Autodesk Inventor part; units mm, degrees
ref_plane "YZ Plane" through (0, 0, 0) normal (1, 0, 0) x (0, 1, 0)
ref_plane "XZ Plane" through (0, 0, 0) normal (0, 1, 0) x (-1, 0, 0)
ref_plane "XY Plane" through (0, 0, 0) normal (0, 0, 1) x (1, 0, 0)
sketch "Sketch1" plane through (0, 0, 0) normal (0, 1, 0) x (-1, 0, 0)
  circle A0 centre (0, 0) radius 90
  line L0 (-25, 120) -> (-25, 60)
  line L1 (-25, 60) -> (-145, 60)
  line L2 (-145, 60) -> (-145, 120)
  line L3 (-145, 120) -> (-25, 120)
  line L4 (-25, 90) -> (0, 90)
  line L5 (-65, 131) -> (-38.5, 131)
  line L6 (-38.5, 131) -> (-38.5, 49)
  line L7 (-38.5, 49) -> (-65, 49)
  line L8 (-65, 49) -> (-65, 131)
  line L9 (-38.5, 90) -> (-25, 90) construction
  circle A1 centre (0, 0) radius 150
  line L10 (-25, 30) -> (25, 30)
  line L11 (25, 30) -> (25, 150)
  line L12 (25, 150) -> (-25, 150)
  line L13 (-25, 150) -> (-25, 30)
  line L14 (-25, 30) -> (25, 150) construction
  line L15 (25, 30) -> (-25, 150) construction
  point P0 (-65, 62.2495)
  point P1 (-65, 60)
  point P2 (-67.082, 60)
  point P3 (25, 147.902)
  point P4 (-25, 147.902)
  dimension "d0" = 180
  dimension "d1" = 25
  dimension "d2" = 60
  dimension "d3" = 120
  dimension "d4" = 82
  dimension "d5" = 26.5
  dimension "d7" = 38.5
  dimension "d8" = 300
  dimension "d18" = 50
  dimension "d19" = 120
extrude "Extrusion1" add sketch "Sketch1" against normal blind 6 contours A0 L1 L8 L7 L6 L13 L10 L11 | A0 L11 A1 L1 | L11 L10 L13 L0 A0 | A0 L4 L0 L13 A1 L11 | L1 A1 L3 L8 A0 | A0 L8 L1 | A0 L0 L4 | L8 L3 L6 A0 | A0 L6 L1 L8 | L1 L6 L7 L8 | L0 L1 L6 A0 | A0 L6 L3 L0 | L8 L5 L6 L3 | L3 A1 L13 L6 L5 L8
hole "Hole1" at (65, 0, 131) at (38.5, 0, 131) at (65, 0, 49) at (38.5, 0, 49) direction (0, -1, 0) diameter 5.6 end through all
extrude "Extrusion2" cut sketch "Sketch1" against normal blind 6 contours L11 L10 L13 L0 A0 | A0 L4 L0 L13 A1 L11 | A0 L0 L4
pattern_circular "Circular Pattern1" count 3 over 360 about axis through (0, 0, 0) along (0, -1, 0) of "Hole1", "Extrusion2"
properties part number "TempPart1"
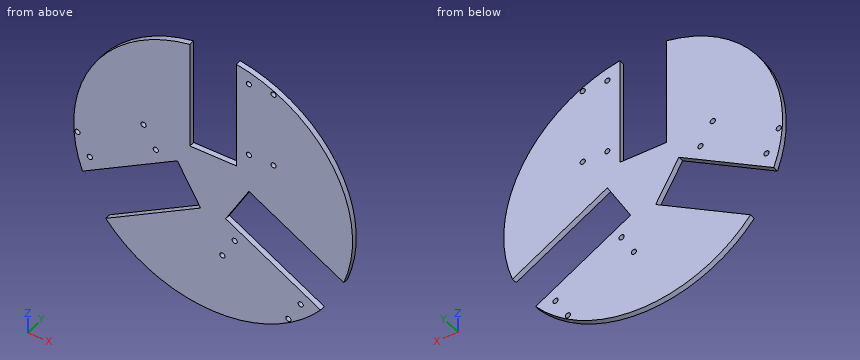
Geometry check sheet. Reference: the model listing, model coordinates, mm. Give positions to 0.01 mm unless a question says otherwise; leave off trailing zeros. Write each loop counter-clockwise with the first axis right and the second up, starting at its lowest first coordinate (ties: lowest second). Pieces come first, ordered by that corner, then holes. Notation, with made-up numbers: (60.25, -15) - (83.25, -15) arc R27 cw to (83.25, 13) - close; hole circle Ø3 at (-5.5, -20). An arc over 180 degrees is marked (long way). Use a Markdown table: item, result.
Q1. Section check A-A, the plane z = 77.5. Enter the section's corners in (x, y).
Computed:
| item | result |
|---|---|
| outline | (-128.43, -6) - (-25, -6) - (-25, 0) - (-128.43, 0) - close; (25, -6) - (128.43, -6) - (128.43, 0) - (25, 0) - close |
Q2. Thickness scan on L1, parallel to Z at x = 38.5, y = -2.9 (1 decimal); L2, parallel to X at y = -4.75, z = -14; L3, parallel to Z at x = -62, y = -0.4. Record the ranges inside material, lowest first. Write a range as [from, to].
Computed:
| item | result |
|---|---|
| L1 | z = [-145, -51.1], [6.6, 46.2], [51.8, 128.2], [133.8, 145] |
| L2 | x = [-149.35, -74.25], [-26.56, 26.56], [74.25, 149.35] |
| L3 | z = [-136.59, -64.66], [-6.93, 6.06], [11.62, 136.59] |
Q3. Section check B-B, the plane x = -87. Enter the section's corners in (y, z).
Computed:
| item | result |
|---|---|
| outline | (-6, -122.19) - (0, -122.19) - (0, -79.1) - (-6, -79.1) - close; (-6, -21.36) - (0, -21.36) - (0, 122.19) - (-6, 122.19) - close |
Q4. Section check D-D, the plane z = 1. Enter the section's corners in (x, y).
Computed:
| item | result |
|---|---|
| outline | (-150, -6) - (-48.27, -6) - (-48.27, 0) - (-150, 0) - close; (-35.22, -6) - (35.22, -6) - (35.22, 0) - (-35.22, 0) - close; (48.27, -6) - (150, -6) - (150, 0) - (48.27, 0) - close |
Q5. Section check C-C, the plane y = -1.1. Give the number of separate pieces and of enclosed holes in the cut face, then the cut area to 3 significant figures.
Computed:
| item | result |
|---|---|
| separate pieces | 1 |
| enclosed holes | 12 |
| area | 52,500 mm² |
Q6. Go/stop test with flat-tipped pins: P1, Ø5, axis at x = 80.95, z = -121.79, coming from the -Y side; P2, Ø1.5, axis at y = -2, z = 58.5, coming from the -X side; P3, Ø1.8, axis at y = -4, z = 84.5, coming from the +X side. Record where each tip stops, or that it passes through.
Computed:
| item | result |
|---|---|
| P1 | passes through |
| P2 | stops at x = -138.44 |
| P3 | stops at x = 124.54 |
